CAD build for the part. Positions are in the model's coordinates, mm. Round coordinates to 2 decimals unless told otherwise and drop trailing zeros. Write each loop counter-clockwise with the first axis right and the second up, starting at its lowest first coordinate (ties: lowest second). Pieces come first, ordered by that corner, then holes. Notation, with made-up numbers: (17, -14) - (23, -14) arc R28 cw to (23, 18) - close; hole circle Ø6 at (-8.5, 65.25). An arc over 180 degrees is marked (long way). Use one line per item in the form item = value. Start each with the question number.
Item 1: Pin check, flat tips, straight feed: pin 1 (3 mm diameter, centred on x = 0, z = 6.5, fed in from +Y); pin 2 (3 mm diameter, centred on x = -1, y = -1.5, fed in from +Z); pin 3 (2 mm diameter, centred on x = -2.5, y = -2.5, fed in from -Z). Stop position of each tip, or through.
Item 2: Band-saw the part on B-B, the plane z = 3.75. List the corners of the cut face in (x, y), and give its area (3 significant figures).
Item 3: Drill centre lines: L1, parallel to Z at x = -3.25, y = 0; L2, parallel to Z at x = -2.25, y = 3; L3, parallel to Z at x = 1.25, y = -0.75. Where is each one in solid material? Low to high.
Item 4: Pull direction Z, two halves, no side cores. Call faces 1 (the cylindrical face through (-0.3, -0.95, -1.2)), 2 (the flat face through (1, -1, 10.008)), 3 (the flat face through (0, 0, -1.397)): +Z half, -Z half, draft (parallel to the pull), parting line (faces both ways), or undercut.
Item 5: Band-saw the part on A-A, the plane z = 12.5. List the corners of the cut face in (x, y), and give its area (3 significant figures).
from build123d import *

# Parameters (mm, degrees)
SKETCH3_R          = 10.452405385
CUT_EXTRUDE1_DEPTH = 20.505116436


with BuildPart() as part:
    # Sketch2 → Revolve1 (revolve)
    with BuildSketch(Plane(origin=(0, 0, 0), x_dir=(0, 0, -1), z_dir=(1, 0, 0)), mode=Mode.PRIVATE) as revolve1_sk:
        with BuildLine():
            Line((-10.0076, 1.7446625), (-10.0076, 1.2461875))
            Line((-10.0076, 1.2461875), (-10.7569, 1.2461875))
            Line((-10.7569, 1.2461875), (-10.7569, 0.99695))
            Line((-10.7569, 0.99695), (-12.2555, 1.7446625))
            Line((-12.2555, 1.7446625), (-12.2555, 1.495425))
            Line((-12.2555, 1.495425), (-13.0048, 1.495425))
            ThreePointArc((-13.0048, 1.495425), (-15.4054584, 1.832401568), (-16.9926, 0))
            Line((-16.9926, 0), (-9.666659115, 0))
            Line((-9.666659115, 0), (18.3896, 0))
            Line((18.3896, 0), (17.891125, 0.99695))
            Line((17.891125, 0.99695), (1.397, 0.99695))
            Line((1.397, 0.99695), (1.016, 0.99695))
            Line((1.016, 0.99695), (1.016, 1.099038642))
            ThreePointArc((1.016, 1.099038642), (1.294911358, 1.37795), (1.397, 1.75895))
            ThreePointArc((1.397, 1.75895), (1.028829656, 3.340753354), (0, 4.5974))
            Line((0, 4.5974), (0, 1.7446625))
            Line((0, 1.7446625), (-10.0076, 1.7446625))
        make_face()
    revolve(revolve1_sk.sketch.rotate(Axis((0, 0, 9.666659115), (0, 0, -1)), 180), axis=Axis((0, 0, 9.666659115), (0, 0, -1)))

    # Sketch3 → Cut-Extrude1 (cut, through all)
    with BuildSketch(Plane.XY.offset(-1.397)):
        Circle(SKETCH3_R)
    extrude(amount=-CUT_EXTRUDE1_DEPTH, mode=Mode.SUBTRACT)


solid = part.part
Determined:
q1.pin_1 = 1.74
q1.pin_2 = 16.91
q1.pin_3 = -1.31
q2.outline = circle Ø3.49 at (0, 0)
q2.area = 9.56 mm²
q3.L1 = -1.07 to 0
q3.L2 = -0.79 to 0
q3.L3 = -1.33 to 10.01, 11.68 to 16.07
q4.face_1 = draft
q4.face_2 = undercut
q4.face_3 = -Z half
q5.outline = circle Ø2.99 at (0, 0)
q5.area = 7.03 mm²
